from build123d import *

# Parameters (mm, degrees)
F1_DEPTH = 3.5
F2_R     = 3.5
F3_DEPTH = 6
F4_R     = 1.5
F5_DEPTH = 29.001


with BuildPart() as f1:
    # F0 (on Top) → F1 (new body, symmetric)
    with BuildSketch(Plane.XY):
        with BuildLine():
            Line((0, -1.75), (0, 0))
            Line((0, 0), (33.5, 0))
            ThreePointArc((33.5, 0), (33.8535533906, 0.1464466094), (34, 0.5))
            Line((34, 0.5), (34, 11.35))
            ThreePointArc((34, 11.35), (34.1903805922, 11.8096194078), (34.65, 12))
            Line((34.65, 12), (34.85, 12))
            ThreePointArc((34.85, 12), (35.3096194078, 11.8096194078), (35.5, 11.35))
            Line((35.5, 11.35), (35.5, -1.75))
            Line((35.5, -1.75), (34.1035533906, -1.75))
            ThreePointArc((34.1035533906, -1.75), (33.8725835075, -1.9043291419), (33.9267766953, -2.1767766953))
            Line((33.9267766953, -2.1767766953), (36.6767766953, -4.9267766953))
            ThreePointArc((36.6767766953, -4.9267766953), (36.7578825325, -4.9809698831), (36.8535533906, -5))
            Line((36.8535533906, -5), (38.85, -5))
            ThreePointArc((38.85, -5), (39.3096194078, -4.8096194078), (39.5, -4.35))
            Line((39.5, -4.35), (39.5, -3.9))
            ThreePointArc((39.5, -3.9), (39.6903805922, -3.4403805922), (40.15, -3.25))
            Line((40.15, -3.25), (40.35, -3.25))
            ThreePointArc((40.35, -3.25), (40.8096194078, -3.0596194078), (41, -2.6))
            Line((41, -2.6), (41, 1.6))
            ThreePointArc((41, 1.6), (40.8096194078, 2.0596194078), (40.35, 2.25))
            Line((40.35, 2.25), (40.15, 2.25))
            ThreePointArc((40.15, 2.25), (39.6903805922, 2.0596194078), (39.5, 1.6))
            Line((39.5, 1.6), (39.5, -1.1))
            ThreePointArc((39.5, -1.1), (39.3096194078, -1.5596194078), (38.85, -1.75))
            Line((38.85, -1.75), (37.5, -1.75))
            Line((37.5, -1.75), (37.5, 11.96))
            ThreePointArc((37.5, 11.96), (37.5117157288, 11.9882842712), (37.54, 12))
            Line((37.54, 12), (82, 12))
            Line((82, 12), (82, 18))
            Line((82, 18), (-19, 18))
            Line((-19, 18), (-19, 12))
            Line((-19, 12), (-12, 12))
            Line((-12, 12), (-12, -4.35))
            ThreePointArc((-12, -4.35), (-11.8096194078, -4.8096194078), (-11.35, -5))
            Line((-11.35, -5), (-0.3535533906, -5))
            ThreePointArc((-0.3535533906, -5), (-0.2578825325, -4.9809698831), (-0.1767766953, -4.9267766953))
            Line((-0.1767766953, -4.9267766953), (2.5732233047, -2.1767766953))
            ThreePointArc((2.5732233047, -2.1767766953), (2.6274164925, -1.9043291419), (2.3964466094, -1.75))
            Line((2.3964466094, -1.75), (0, -1.75))
        make_face()
    extrude(amount=F1_DEPTH, both=True)

    # F2 (on face) → F3 (join)
    with BuildSketch(Plane(origin=(0, 18, 0), x_dir=(-1, 0, 0), z_dir=(0, 1, 0))):
        with Locations((-78.5, 0)):
            Circle(F2_R)
        with Locations((15.5, 0)):
            Circle(F2_R)
    extrude(amount=F3_DEPTH)

    # F4 (on face) → F5 (cut, through all)
    with BuildSketch(Plane(origin=(0, 24, 0), x_dir=(-1, 0, 0), z_dir=(0, 1, 0))):
        with Locations((-78.5, 0)):
            Circle(F4_R)
        with Locations((15.5, 0)):
            Circle(F4_R)
    extrude(amount=-F5_DEPTH, mode=Mode.SUBTRACT)


solid = f1.part
Work out the finished part from the listing and answer in its coordinate system (mm). A direction names the side the tool comes from. Round coordinates to 2 decimals unless told otherwise and drop trailing zeros. Write each loop counter-clockwise with the first axis right and the second up, starting at its lowest first coordinate (ties: lowest second). Pieces come first, ordered by that corner, then holes. Notation, with made-up numbers: M -27,-27 L 28,-27 A12 cw 28,-20 Z; hole C -21,-25.5 d3. An arc over 180 degrees is marked long. Use a Markdown table: item, result.
1) Determine the mould class of faces 1 (the face through (-14, 18, 0)), 2 (the face through (-18.84, 20.96, 1.05)), 3 (the face through (1.18, -3.57, 0.05)) for opening direction Z: pulls with the +Z half, pulls with the -Z half, needs draft (parallel to the pull), parting line crosses it, or undercut.
Taken from the geometry:
| item | result |
|---|---|
| face 1 | undercut |
| face 2 | parting line crosses it |
| face 3 | needs draft |
2) Which of the six approach directions +Z, -Z, +X, -X, +Y, -Y give full straight-line access (tool end or side, diameter ignored) to faces 4 (the face through (81, 18, -3)), 5 (the face through (-16, 12, -2)), 6 (the face through (0, -1, 0)), 7 (the face through (-18, 18, -3)), 8 (the face through (81, 18, 3))?
Taken from the geometry:
| item | result |
|---|---|
| face 4 | -Z, +X, +Y |
| face 5 | +Z, -Z, -X, -Y |
| face 6 | +Z, -Z |
| face 7 | -Z, -X, +Y |
| face 8 | +Z, +X, +Y |
3) The part is cut by section B-B on x = 10. Give the vertices of the cut face in (y, z).
Taken from the geometry:
| item | result |
|---|---|
| outline | M 0,-3.5 L 18,-3.5 L 18,3.5 L 0,3.5 Z |
4) The part is cut by section C-C on x = 45.5. Give the vertices of the cut face in (y, z), plus the area to 3 significant figures.
Taken from the geometry:
| item | result |
|---|---|
| outline | M 12,-3.5 L 18,-3.5 L 18,3.5 L 12,3.5 Z |
| area | 42.0 mm2 |
5) Flat-ended cylindrical pins translate along their axes: pin 1 (2 mm diameter, centred on x = -17, z = -1, fed in from -Y); pin 2 (3.5 mm diameter, centred on y = 7, z = 1, fed in from +X); pin 3 (1.9 mm diameter, centred on x = 1.5, z = -1, fed in from +Y). Find the tip coordinate at first contact, or state that the pin passes through.
Taken from the geometry:
| item | result |
|---|---|
| pin 1 | stops at y = 12 |
| pin 2 | stops at x = 37.5 |
| pin 3 | stops at y = 18 |
6) The part is cut by section A-A on y = 16. Give the vertices of the cut face in (x, z).
Taken from the geometry:
| item | result |
|---|---|
| outline | M -19,-3.5 L 82,-3.5 L 82,3.5 L -19,3.5 Z; hole C -15.5,0 d3; hole C 78.5,0 d3 |
7) Consider line 1 (X direction, y = 9.5, z = -1.75); line 2 (Y direction, x = 38.5, z = 1.75); line 3 (Z direction, x = -15.5, y = 18.5). Determine where each line is inside the solid, lowest interval first. Write a range as [from, to].
Taken from the geometry:
| item | result |
|---|---|
| line 1 | x = [-12, 34], [35.5, 37.5] |
| line 2 | y = [-5, -1.75], [12, 18] |
| line 3 | z = [-3.5, -1.5], [1.5, 3.5] |
